Check sheet for the drawn part. Datum: minimum x, y, z corner. Units: mm. A direction names the side the tool comes from. Round coordinates to 2 decimals unless told otherwise and drop trailing zeros. Order: outer loops, then holes, each group sorted by start corner. A loop starts at its lowest first (then second) coordinate and runs counter-clockwise, first axis right, second up. Notation, with made-up numbers: M -0.5,52 L 20.5,52 A23 cw 20.5,62 Z; hole C 21.5,67 d10. An arc over 180 degrees is marked long. Use one line per item in the form item = value. Start each with the question number.
Item 1: Cross-section at C-C on z = 1. Enter the section's corners in (x, y).
Item 2: Release check for a two-part mould opening along X. For the marked faces 1, 2 and 3 record: +X half, -X half, draft (parallel to the pull), parting line (faces both ways), or undercut.
Item 3: Cross-section at D-D on y = 37. Enter the section's corners in (x, z).
Item 4: Cross-section at A-A on y = 25. Enter the section's corners in (x, z), then the cut area to 3 significant figures.
Item 5: Tool access check on the marked faces 4 and 5. Record the directions out of +Z, -Z, +X, -X, +Y, -Y that give a thin tool (end or side, any length) a straight path to the whole face; none if there is none.
Item 6: Go/stop test with flat-tipped pins: pin 1 Ø1 at (x, z) = (31.5, 1) entering from -Y; pin 2 Ø1.5 at (x, z) = (35.5, 7) entering from +Y; pin 3 Ø3 at (x, y) = (18.5, 19) entering from +Z. Record where each tip stops, or that it passes through.
Item 7: Thickness scan on probe 1 along Y at (x, z) = (25, 5.4); probe 2 along Y at (x, z) = (25, 0.55); probe 3 along Z at (x, y) = (32.5, 32). Record the ranges inside material, lowest first. Write a range as [from, to].
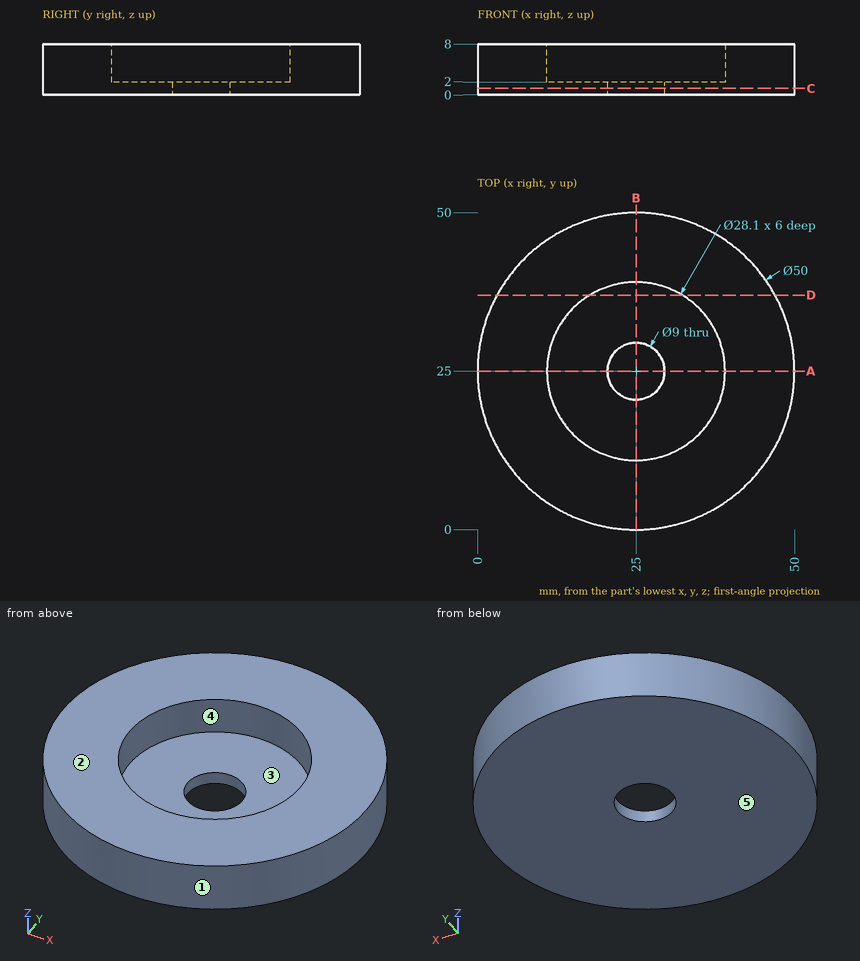
Output values:
q1.outline = C 25,25 d50; hole C 25,25 d9
q2.face_1 = parting line
q2.face_2 = draft
q2.face_3 = undercut
q3.outline = M 3.07,0 L 46.93,0 L 46.93,8 L 32.31,8 L 32.31,2 L 17.69,2 L 17.69,8 L 3.07,8 Z
q4.outline = M 0,0 L 20.5,0 L 20.5,2 L 10.95,2 L 10.95,8 L 0,8 Z; M 29.5,0 L 50,0 L 50,8 L 39.05,8 L 39.05,2 L 29.5,2 Z
q4.area = 213 mm2
q5.face_4 = +Z
q5.face_5 = -Z, +X, -X, +Y, -Y
q6.pin_1 = 0.73
q6.pin_2 = 48.02
q6.pin_3 = 2
q7.probe_1 = [0, 10.95], [39.05, 50]
q7.probe_2 = [0, 20.5], [29.5, 50]
q7.probe_3 = [0, 2]
